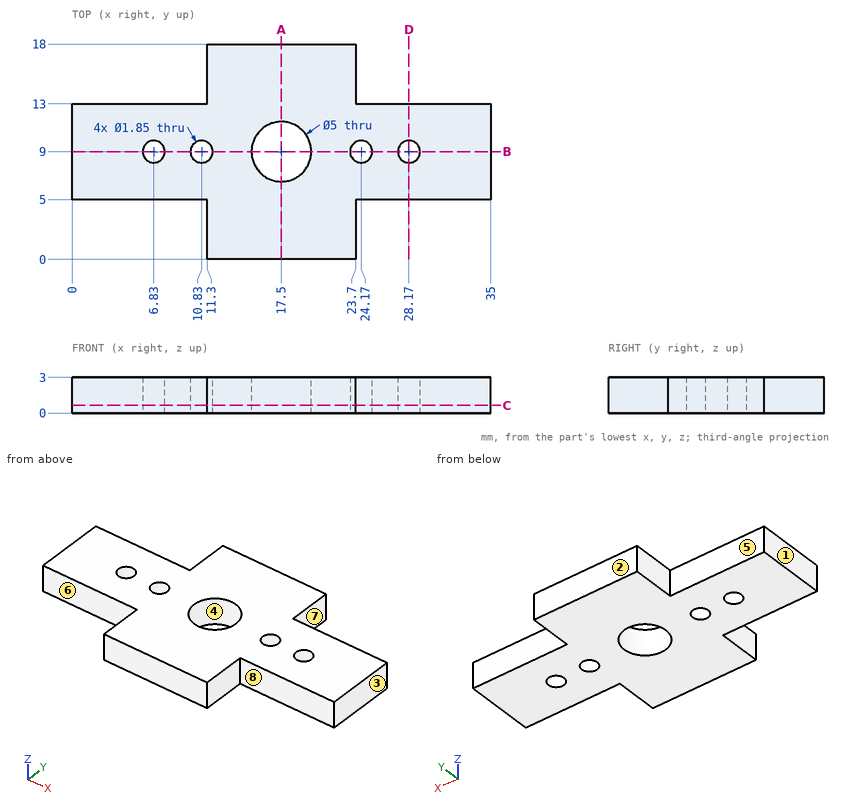
Input: dimensioned drawing with shaded views. Units: mm. Origin: part minimum x, y, z. A direction names the side the tool comes from. Coordinates: 2 decimals unless noted, no trailing zeros. Write each loop counter-clockwise with the first axis right and the second up, starting at its lowest first coordinate (ties: lowest second). Pieces come first, ordered by that corner, then holes. Notation, with made-up numbers: M 40.5,-7 L 93.5,-7 A29 cw 93.5,21 Z; hole C -21,36 d1. An arc over 180 degrees is marked long. Answer as a JSON object with one key per item and string values. Group by question number.
(1) Set-up query: the marked faces 5, 6, 7 and 8. Return all of +Z, -Z, +X, -X, +Y, -Y with unobstructed straight access to the full face (end or side cutting, diameter ignored); none if empty.
(2) Section C-C on z = 0.65. Output: boundary loops of the cut face in (x, y) (3 decimals).
(3) Ray query, line 1 along X through (y, z) = (8.75, 0.45); line 2 along Y through (x, z) = (6.83, 2.25) (3 decimals); line 3 along X through (y, z) = (9.5, 2.45). Return the intervals inside material, ascending. Write a range as [from, to].
(4) Section A-A on x = 17.5. Output: boundary loops of the cut face in (y, z), plus the area to 3 significant figures.
(5) Section D-D on x = 28.17. Output: boundary loops of the cut face in (y, z) (3 decimals).
(6) Contact query for flat-ended pins moving along their axis: P1, Ø1.7, axis at x = 28.17, y = 9, coming from the +Z side; P2, Ø6, axis at x = 13, y = 11.5, coming from the -Z side; P3, Ø1.5, axis at x = 30, z = 1.5, coming from the +Y side; P4, Ø1.5, axis at y = 14.5, z = 1.5, coming from the -X side. Output: stop coordinate, or through.
(7) Mould query, pull axis X, two halves, no side actions, for the marked faces 1, 2, 3 and 4. Classes: pulls with the +X half, pulls with the -X half, needs draft (parallel to the pull), parting line crosses it, or undercut.
(8) Section B-B on y = 9. Output: boundary loops of the cut face in (x, z) (3 decimals).
Result set:
{
 "1": {"face 5": "+Z, -Z, -X, +Y", "face 6": "+Z, -Z, -X, -Y", "face 7": "+Z, -Z, +X, +Y", "face 8": "+Z, -Z, +X, -Y"},
 "2": {"outline": "M 0,5 L 11.3,5 L 11.3,0 L 23.7,0 L 23.7,5 L 35,5 L 35,13 L 23.7,13 L 23.7,18 L 11.3,18 L 11.3,13 L 0,13 Z; hole C 6.83,9 d1.85; hole C 10.83,9 d1.85; hole C 17.5,9 d5; hole C 24.17,9 d1.85; hole C 28.17,9 d1.85"},
 "3": {"line 1": "x = [0, 5.94], [7.72, 9.94], [11.72, 15.01], [19.99, 23.28], [25.06, 27.28], [29.06, 35]", "line 2": "y = [5, 8.075], [9.925, 13]", "line 3": "x = [0, 6.05], [7.61, 10.05], [11.61, 15.05], [19.95, 23.39], [24.95, 27.39], [28.95, 35]"},
 "4": {"outline": "M 0,0 L 6.5,0 L 6.5,3 L 0,3 Z; M 11.5,0 L 18,0 L 18,3 L 11.5,3 Z", "area": "39.0 mm2"},
 "5": {"outline": "M 5,0 L 8.075,0 L 8.075,3 L 5,3 Z; M 9.925,0 L 13,0 L 13,3 L 9.925,3 Z"},
 "6": {"P1": "passes through", "P2": "stops at z = 0", "P3": "stops at y = 13", "P4": "stops at x = 11.3"},
 "7": {"face 1": "pulls with the -X half", "face 2": "needs draft", "face 3": "pulls with the +X half", "face 4": "undercut"},
 "8": {"outline": "M 0,0 L 5.905,0 L 5.905,3 L 0,3 Z; M 7.755,0 L 9.905,0 L 9.905,3 L 7.755,3 Z; M 11.755,0 L 15,0 L 15,3 L 11.755,3 Z; M 20,0 L 23.245,0 L 23.245,3 L 20,3 Z; M 25.095,0 L 27.245,0 L 27.245,3 L 25.095,3 Z; M 29.095,0 L 35,0 L 35,3 L 29.095,3 Z"}
}
